Geometry: see drawing. Coordinates: mm, zero at the bounding-box minimum. A direction names the side the tool comes from. Coordinates: 2 decimals unless noted, no trailing zeros. Write each loop counter-clockwise with the first axis right and the second up, starting at its lowest first coordinate (ties: lowest second). Pieces come first, ordered by that corner, then holes. Notation, with made-up numbers: (-25, -2) - (1, -2) arc R22 ccw to (1, 8) - close; hole circle Ø8 at (30, 4.25). An arc over 180 degrees is marked (long way). One line per question, with ' | ' between items. Start each with the question number.
Q1. Access query for the marked faces 1 and 2. Directions: +Z, -Z, +X, -X, +Y, -Y. A direction counts if a zero-diameter tool reaches every point of the face in a straight line with its end or side. Return the directions, or none.
Q2. Line query: line 1 (Y direction, x = 5.5, z = 3.75); line 2 (Y direction, x = 5.5, z = 3.45); line 3 (Z direction, x = 2, y = 4.5). Output: solid intervals per line, ascending.
Q3. Cut plane A-A, the plane z = 2.5. Return loops of the section in (x, y), plus the area to 3 significant figures.
Q4. Draft query along X for the marked faces 3, 4 and 5. Return one class per face: +X half, -X half, draft (parallel to the pull), parting line (faces both ways), or undercut.
Q5. Contact query for flat-ended pins moving along their axis: P1, Ø3, axis at x = 6.5, y = 1.5, coming from the +Z side; P2, Ø1.5, axis at x = 10, z = 0.5, coming from the +Y side; P3, Ø1, axis at y = 2, z = 0.5, coming from the +X side. Output: stop coordinate, or through.
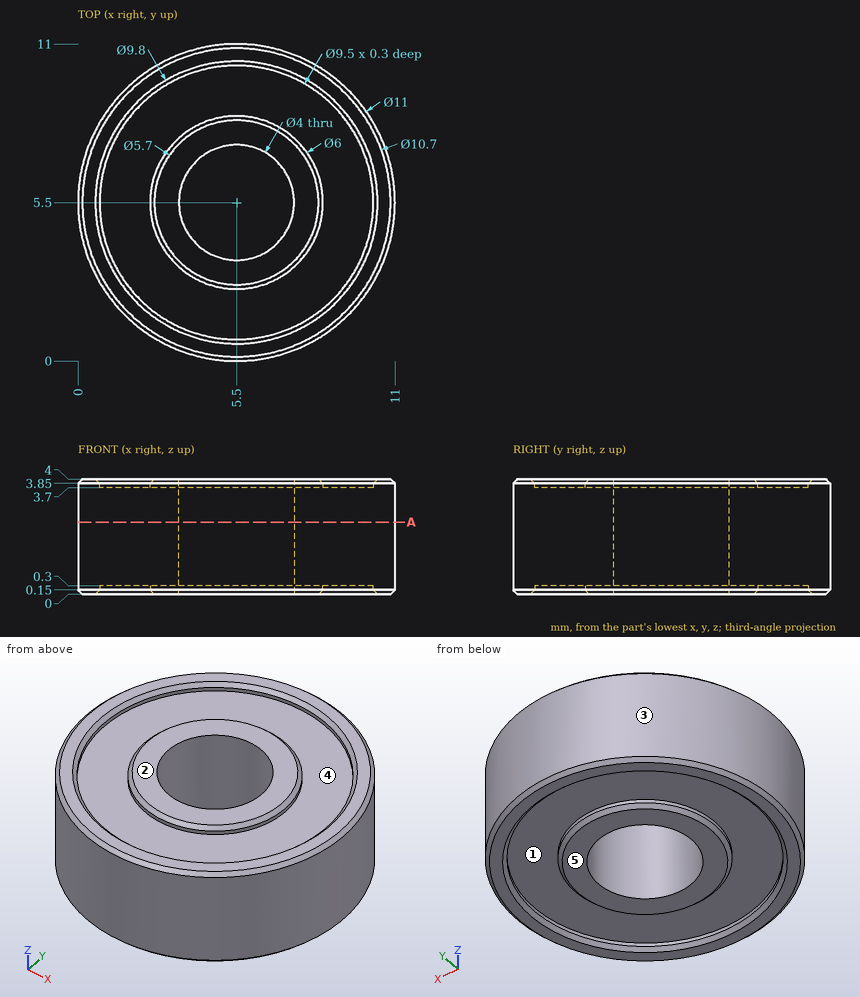
Reply:
1) face 1: -Z | face 2: +Z, +X, -X, +Y, -Y
2) line 1: y = 0 to 0.75, 2.5 to 3.5, 7.5 to 8.5, 10.25 to 11 | line 2: y = 0 to 3.5, 7.5 to 11 | line 3: z = 0.3 to 3.7
3) outline: circle Ø11 at (5.5, 5.5); hole circle Ø4 at (5.5, 5.5) | area: 82.5 mm^2
4) face 3: parting line | face 4: undercut | face 5: draft
5) P1: stops at z = 4 | P2: stops at y = 9.52 | P3: stops at x = 10.11
